```python
from build123d import *

# Parameters (mm, degrees)
SKETCH9_W               = 50
SKETCH9_H               = 50
SKETCH9_R               = 3.75
SKETCH9_R_2             = 1.5
BOSS_EXTRUDE2_DEPTH     = 2
BOSS_EXTRUDE3_DEPTH     = 20
SKETCH12_R              = 2
CUT_EXTRUDE1_DEPTH      = 2
CUT_EXTRUDE2_DEPTH      = 50
CUT_EXTRUDE2_DEPTH_BACK = 2
SKETCH13_R              = 2
SKETCH15_W              = 50
SKETCH15_H              = 15
BOSS_EXTRUDE4_DEPTH     = 2
CUT_EXTRUDE4_DEPTH      = 2
BOSS_EXTRUDE7_START     = 2
BOSS_EXTRUDE7_DEPTH     = 2
BOSS_EXTRUDE8_START     = 2
BOSS_EXTRUDE8_DEPTH     = 2
SKETCH17_W              = 50
SKETCH17_H              = 2
BOSS_EXTRUDE5_DEPTH     = 20
SKETCH19_R              = 2
CUT_EXTRUDE5_DEPTH      = 49
SKETCH20_W              = 2
SKETCH20_H              = 13
BOSS_EXTRUDE6_DEPTH     = 20
FILLET2_R               = 2
FILLET3_R               = 2
FILLET5_R               = 2
FILLET6_R               = 2
FILLET7_R               = 2
FILLET8_R               = 2
FILLET9_R               = 2
FILLET10_R              = 2


with BuildPart() as part:
    # Sketch9 → Boss-Extrude2 (new body)
    with BuildSketch(Plane.XY):
        with Locations((25, 25)):
            Rectangle(SKETCH9_W, SKETCH9_H)
        with Locations((25, 35)):
            Circle(SKETCH9_R, mode=Mode.SUBTRACT)
        with Locations((16.4, 35)):
            Circle(SKETCH9_R_2, mode=Mode.SUBTRACT)
        with Locations((33.6, 35)):
            Circle(SKETCH9_R_2, mode=Mode.SUBTRACT)
        with BuildLine():
            Line((9, 9.5), (9, 10.5))
            ThreePointArc((9, 10.5), (7, 12.5), (5, 10.5))
            Line((5, 10.5), (5, 9.5))
            ThreePointArc((5, 9.5), (7, 7.5), (9, 9.5))
        make_face(mode=Mode.SUBTRACT)
        with BuildLine():
            Line((45, 9.5), (45, 10.5))
            ThreePointArc((45, 10.5), (43, 12.5), (41, 10.5))
            Line((41, 10.5), (41, 9.5))
            ThreePointArc((41, 9.5), (43, 7.5), (45, 9.5))
        make_face(mode=Mode.SUBTRACT)
    extrude(amount=BOSS_EXTRUDE2_DEPTH)

    # Sketch11 → Boss-Extrude3 (add)
    with BuildSketch(Plane(origin=(0, 0, 0), x_dir=(-1, 0, 0), z_dir=(0, 0, -1))):
        Polygon((-48, 22), (-48, 50), (-50, 50), (-50, 20), (-28.5, 20), (-28.5, 22), align=None)
        Polygon((-7, 20), (0, 20), (0, 50), (-2, 50), (-2, 22), (-21.5, 22), (-21.5, 20), align=None)
    extrude(amount=BOSS_EXTRUDE3_DEPTH)

    # Sketch12 → Cut-Extrude1 (cut)
    with BuildSketch(Plane(origin=(0, 22, 0), x_dir=(1, 0, 0), z_dir=(0, 1, 0))):
        with Locations(Location((38.5, 10, 0), (0, 0, 180))):
            Circle(SKETCH12_R)
    extrude(amount=-CUT_EXTRUDE1_DEPTH, mode=Mode.SUBTRACT)

    # Sketch13 → Cut-Extrude2 (cut, two sides: drawn at the far end of the back side and taken through both)
    with BuildSketch(Plane(origin=(0, 22, 0), x_dir=(1, 0, 0), z_dir=(0, 1, 0)).offset(-CUT_EXTRUDE2_DEPTH_BACK)):
        with Locations(Location((11.5, 10, 0), (0, 0, 270))):
            Circle(SKETCH13_R)
    extrude(amount=CUT_EXTRUDE2_DEPTH + CUT_EXTRUDE2_DEPTH_BACK, mode=Mode.SUBTRACT)

    # Sketch15 → Boss-Extrude4 (add)
    with BuildSketch(Plane.XY.offset(2)):
        with Locations((25, 57.5)):
            Rectangle(SKETCH15_W, SKETCH15_H)
        with BuildLine():
            ThreePointArc((27.004582083, 57.912478056), (29.731698949, 54.662426734), (26.481647627, 51.935309868))
            ThreePointArc((26.481647627, 51.935309868), (25, 52), (23.518352373, 51.935309868))
            ThreePointArc((23.518352373, 51.935309868), (20.268301051, 54.662426734), (22.995417917, 57.912478056))
            ThreePointArc((22.995417917, 57.912478056), (25, 58), (27.004582083, 57.912478056))
        make_face(mode=Mode.SUBTRACT)
    extrude(amount=-BOSS_EXTRUDE4_DEPTH)

    # Sketch15<3> → Cut-Extrude4 (cut)
    with BuildSketch(Plane.XY.offset(2)):
        with BuildLine():
            ThreePointArc((6.101516985, 21.890944362), (10.276413331, 21.13580166), (11.031556032, 25.310698007))
            ThreePointArc((11.031556032, 25.310698007), (10.240231867, 26.564998835), (9.561238449, 27.883495115))
            ThreePointArc((9.561238449, 27.883495115), (5.580897313, 29.352128645), (4.112263784, 25.371787509))
            ThreePointArc((4.112263784, 25.371787509), (5.030901937, 23.5879396), (6.101516985, 21.890944362))
        make_face()
        with BuildLine():
            ThreePointArc((38.925584753, 25.249200582), (39.662311577, 21.07101514), (43.840497019, 21.807741964))
            ThreePointArc((43.840497019, 21.807741964), (44.918584287, 23.5), (45.845079102, 25.27977998))
            ThreePointArc((45.845079102, 25.27977998), (44.394010526, 29.266558126), (40.40723238, 27.81548955))
            ThreePointArc((40.40723238, 27.81548955), (39.722431864, 26.5), (38.925584753, 25.249200582))
        make_face()
    extrude(amount=-CUT_EXTRUDE4_DEPTH, mode=Mode.SUBTRACT)

    # Sketch21 → Boss-Extrude7 (add)
    with BuildSketch(Plane.XY.offset(BOSS_EXTRUDE7_START)):
        with BuildLine():
            Line((43.964469864, 22), (38.801611908, 22))
            ThreePointArc((38.801611908, 22), (41.268659486, 20.530652583), (43.840497019, 21.807741964))
            ThreePointArc((43.840497019, 21.807741964), (43.90431667, 21.90268887), (43.964469864, 22))
        make_face()
    extrude(amount=-BOSS_EXTRUDE7_DEPTH)

    # Sketch24 → Boss-Extrude8 (add)
    with BuildSketch(Plane.XY.offset(BOSS_EXTRUDE8_START)):
        with BuildLine():
            ThreePointArc((6.101516985, 21.890944362), (8.631925352, 20.601533886), (11.103734084, 22))
            Line((11.103734084, 22), (6.029338933, 22))
            ThreePointArc((6.029338933, 22), (6.064833637, 21.945078831), (6.101516985, 21.890944362))
        make_face()
    extrude(amount=-BOSS_EXTRUDE8_DEPTH)

    # Sketch17 → Boss-Extrude5 (add)
    with BuildSketch(Plane(origin=(0, 0, 0), x_dir=(-1, 0, 0), z_dir=(0, 0, -1))):
        with Locations((-25, 64)):
            Rectangle(SKETCH17_W, SKETCH17_H)
    extrude(amount=BOSS_EXTRUDE5_DEPTH)

    # Sketch19 → Cut-Extrude5 (cut)
    with BuildSketch(Plane(origin=(0, 65, 0), x_dir=(1, 0, 0), z_dir=(0, 1, 0))):
        with Locations(Location((38.5, 10, 0), (0, 0, 180))):
            Circle(SKETCH19_R)
        with Locations(Location((11.5, 10, 0), (0, 0, 270))):
            Circle(SKETCH19_R)
    extrude(amount=-CUT_EXTRUDE5_DEPTH, mode=Mode.SUBTRACT)

    # Sketch20 → Boss-Extrude6 (add)
    with BuildSketch(Plane(origin=(0, 0, 0), x_dir=(-1, 0, 0), z_dir=(0, 0, -1))):
        with Locations((-49, 56.5)):
            Rectangle(SKETCH20_W, SKETCH20_H)
        with Locations((-1, 56.5)):
            Rectangle(SKETCH20_W, SKETCH20_H)
    extrude(amount=BOSS_EXTRUDE6_DEPTH)

    # Fillet2
    fillet2_edges = [part.edges().sort_by_distance(p)[0] for p in [
        (0, 65, -9),
    ]]
    fillet(fillet2_edges, radius=FILLET2_R)

    # Fillet3
    fillet3_edges = [part.edges().sort_by_distance(p)[0] for p in [
        (50, 65, -9),
    ]]
    fillet(fillet3_edges, radius=FILLET3_R)

    # Fillet5
    fillet5_edges = [part.edges().sort_by_distance(p)[0] for p in [
        (50, 20, -10),
    ]]
    fillet(fillet5_edges, radius=FILLET5_R)

    # Fillet6
    fillet6_edges = [part.edges().sort_by_distance(p)[0] for p in [
        (0, 20, -10),
    ]]
    fillet(fillet6_edges, radius=FILLET6_R)

    # Fillet7
    fillet7_edges = [part.edges().sort_by_distance(p)[0] for p in [
        (48, 63, -10),
    ]]
    fillet(fillet7_edges, radius=FILLET7_R)

    # Fillet8
    fillet8_edges = [part.edges().sort_by_distance(p)[0] for p in [
        (2, 22, -10),
    ]]
    fillet(fillet8_edges, radius=FILLET8_R)

    # Fillet9
    fillet9_edges = [part.edges().sort_by_distance(p)[0] for p in [
        (2, 63, -10),
    ]]
    fillet(fillet9_edges, radius=FILLET9_R)

    # Fillet10
    fillet10_edges = [part.edges().sort_by_distance(p)[0] for p in [
        (48, 22, -10),
    ]]
    fillet(fillet10_edges, radius=FILLET10_R)


solid = part.part
```
The model under review builds one solid part; all positions refer to its coordinate system, in mm. A direction names the side the tool comes from. Give positions to 0.01 mm unless a question says otherwise; leave off trailing zeros. Loops run counter-clockwise (first coordinate to the right, second up) from the corner with the lowest first, then second, coordinate; pieces in that order, holes last. Notation, with made-up numbers: (78, 30) - (86, 30) arc R23 cw to (86, 63) - close; hole circle Ø11 at (42, -4.5). An arc over 180 degrees is marked (long way). Answer as a JSON object with one key per item and string values.
Q1. Insertion check: pin 1 (0.6 mm diameter, centred on y = 20.5, z = -12.5, fed in from +X); pin 2 (6 mm diameter, centred on x = 36.5, z = -10, fed in from -Y); pin 3 (4 mm diameter, centred on x = 29, y = 44, fed in from -Z). Each pin has a flat end and moves straight along its axis. Give the tip position at first contact, or say it passes through.
Worked out:
{"pin 1": "stops at x = 49.6", "pin 2": "stops at y = 20", "pin 3": "stops at z = 0"}
Q2. Add section D-D on x = 43. State the section outline as (y, z) points.
Worked out:
{"outline": "(0, 0) - (7.5, 0) - (7.5, 2) - (0, 2) - close; (12.5, 0) - (20, 0) - (20, -20) - (22, -20) - (22, 2) - (12.5, 2) - close; (29.54, 0) - (63, 0) - (63, -20) - (65, -20) - (65, 2) - (29.54, 2) - close"}
Q3. For faces 4 (the cylindrical face through (49.43, 20.6, -10.14)), 5 (the flat face through (28.5, 21, -10)), 6 (the cylindrical face through (7, 7.5, 1)), list the 3-axis set-ups (+Z, -Z, +X, -X, +Y, -Y) from which the entire face can be reached by the end or side of a thin tool; tool diameter is ignored.
Worked out:
{"face 4": "-Z, +X, -Y", "face 5": "-Z, -Y", "face 6": "+Z, -Z"}
Q4. Add section C-C on x = 33.6. State the section outline as (y, z) points.
Worked out:
{"outline": "(0, 0) - (20, 0) - (20, -20) - (22, -20) - (22, 0) - (33.5, 0) - (33.5, 2) - (0, 2) - close; (36.5, 0) - (63, 0) - (63, -20) - (65, -20) - (65, 2) - (36.5, 2) - close"}
Q5. Add section B-B on z = -15. State the section outline as (x, y) points.
Worked out:
{"outline": "(0, 22) arc R2 ccw to (2, 20) - (21.5, 20) - (21.5, 22) - (4, 22) arc R2 cw to (2, 24) - (2, 61) arc R2 cw to (4, 63) - (46, 63) arc R2 cw to (48, 61) - (48, 24) arc R2 cw to (46, 22) - (28.5, 22) - (28.5, 20) - (48, 20) arc R2 ccw to (50, 22) - (50, 63) arc R2 ccw to (48, 65) - (2, 65) arc R2 ccw to (0, 63) - close"}
Q6. To check wall thickness, follow line 1 along Y through (x, z) = (19, -12.5); line 2 along X through (y, z) = (41.5, -15.25); line 3 along Y through (x, z) = (33.6, 1.4). State the ranges of each line that lie inside material, in increasing order.
Worked out:
{"line 1": "y = 20 to 22, 63 to 65", "line 2": "x = 0 to 2, 48 to 50", "line 3": "y = 0 to 33.5, 36.5 to 65"}
Q7. Add section A-A on y = 42. State the section outline as (x, z) points.
Worked out:
{"outline": "(0, -20) - (2, -20) - (2, 0) - (48, 0) - (48, -20) - (50, -20) - (50, 2) - (0, 2) - close"}
Q8. Mouldability with a two-part tool opening along X and no side actions: class faces 1 (the flat face through (50, 38, -9)), 2 (the cylindrical face through (0.57, 64.4, -8.85)), 3 (the cylindrical face through (7, 12.5, 1)) as +X half, -X half, draft (parallel to the pull), parting line (faces both ways), or undercut.
Worked out:
{"face 1": "+X half", "face 2": "-X half", "face 3": "undercut"}
